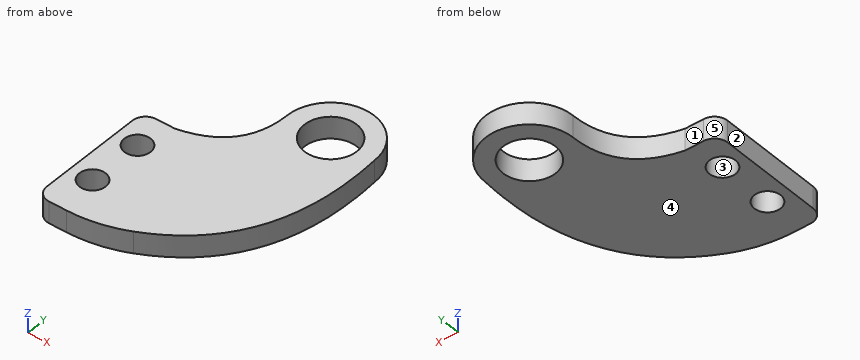
from build123d import *

# Parameters (mm, degrees)
SKETCH1_R           = 3
SKETCH1_R_2         = 6
BOSS_EXTRUDE1_DEPTH = 5
FILLET1_R           = 30
FILLET3_R           = 3
FILLET4_R           = 3


with BuildPart() as part:
    # Sketch1 → Boss-Extrude1 (new body)
    with BuildSketch(Plane.XY):
        with BuildLine():
            Line((685.352484273, 879.16298506), (685.352484273, 849.16298506))
            Line((685.352484273, 849.16298506), (697.448463409, 849.16298506))
            add(Edge.make_bspline(
                [(697.448463409, 849.16298506), (728.616221011, 858.08895863), (725.678478781, 894.611707807)],
                knots=[0, 0, 0, 1, 1, 1], degree=2))
            ThreePointArc((725.678478781, 894.611707807), (715.678478781, 904.611707807), (705.678478781, 894.611707807))
            ThreePointArc((705.678478781, 894.611707807), (705.67849738, 894.592421342), (705.678553175, 894.573134948))
            add(Edge.make_bspline(
                [(705.678553175, 894.573134948), (705.693307068, 881.810970257), (692.631868047, 879.16298506)],
                knots=[0.001508038, 0.001508038, 0.001508038, 1, 1, 1], degree=2))
            Line((692.631868047, 879.16298506), (685.352484273, 879.16298506))
        make_face()
        with Locations((690.448463409, 858.739216263)):
            Circle(SKETCH1_R, mode=Mode.SUBTRACT)
        with Locations((690.448463409, 871.339216263)):
            Circle(SKETCH1_R, mode=Mode.SUBTRACT)
        with Locations((715.678478781, 894.611707807)):
            Circle(SKETCH1_R_2, mode=Mode.SUBTRACT)
    extrude(amount=BOSS_EXTRUDE1_DEPTH)

    # Fillet1
    fillet1_edges = [part.edges().sort_by_distance(p)[0] for p in [
        (697.448463409, 849.16298506, 2.5),
    ]]
    fillet(fillet1_edges, radius=FILLET1_R)

    # Fillet3
    fillet3_edges = [part.edges().sort_by_distance(p)[0] for p in [
        (685.352484273, 879.16298506, 2.5),
    ]]
    fillet(fillet3_edges, radius=FILLET3_R)

    # Fillet4
    fillet4_edges = [part.edges().sort_by_distance(p)[0] for p in [
        (685.352484273, 849.16298506, 2.5),
    ]]
    fillet(fillet4_edges, radius=FILLET4_R)


solid = part.part
The model under review builds one solid part; all positions refer to its coordinate system, in mm. Face numbers are marked on the shaded views. A direction names the side the tool comes from. Round coordinates to 2 decimals unless told otherwise and drop trailing zeros. Loops run counter-clockwise (first coordinate to the right, second up) from the corner with the lowest first, then second, coordinate; pieces in that order, holes last. Notation, with made-up numbers: M -5.75,54 L 4.25,54 A21 cw 4.25,62 Z; hole C -39.75,1.25 d11. An arc over 180 degrees is marked long. Answer as CSV lines item,"result". Start each with the question number.
Item 1: Wall thickness on line 1 (Y direction, x = 689, z = 0.9); line 2 (X direction, y = 869.5, z = 0.5); line 3 (Y direction, x = 714.5, z = 4.8): over which ranges is each line inside the solid? List them lowest first. Write a range as [from, to].
Item 2: Consider section B-B (x = 689.5). Write out the cut boundary in (y, z).
Item 3: Insertion check: P1, Ø2, axis at x = 690.5, z = 2.5, coming from the +Y side; P2, Ø1.5, axis at y = 892.5, z = 3, coming from the +X side; P3, Ø1, axis at y = 893.5, z = 3.5, coming from the +X side. Each pin has a flat end and moves straight along its axis. Give the tip position at first contact, or say it passes through.
Item 4: Mouldability with a two-part tool opening along X and no side actions: class the marked faces 3, 4 and 5 as released by +X, released by -X, zero draft, split by the parting line, or undercut.
Item 5: For the marked faces 1 and 2, list the 3-axis set-ups (+Z, -Z, +X, -X, +Y, -Y) from which the entire face can be reached by the end or side of a thin tool; tool diameter is ignored.
Item 6: Consider section A-A (y = 896). Write out the cut boundary in (x, z).
Item 7: Consider section C-C (z = 1.6). State how many separate pieces and enclosed holes the cut face has, then the cut area to 3 significant figures.
Answer:
1,line 1,"y = [849.16, 856.11], [861.37, 868.71], [873.97, 879.16]"
1,line 2,"x = [685.35, 688.08], [692.82, 722.44]"
1,line 3,"y = [858.24, 888.73], [900.49, 904.54]"
2,outline,"M 849.16,0 L 855.89,0 L 855.89,5 L 849.16,5 Z; M 861.59,0 L 868.49,0 L 868.49,5 L 861.59,5 Z; M 874.19,0 L 879.16,0 L 879.16,5 L 874.19,5 Z"
3,P1,"stops at y = 879.16"
3,P2,"stops at x = 725.86"
3,P3,"stops at x = 725.79"
4,face 3,"undercut"
4,face 4,"zero draft"
4,face 5,"released by -X"
5,face 1,"+Z, -Z, -X, +Y"
5,face 2,"+Z, -Z, -X, +Y, -Y"
6,outline,"M 705.78,0 L 709.84,0 L 709.84,5 L 705.78,5 Z; M 721.52,0 L 725.58,0 L 725.58,5 L 721.52,5 Z"
7,separate pieces,"1"
7,enclosed holes,"3"
7,area,"1,290 mm^2"
